from build123d import *

# Parameters (mm, degrees)
SCHIZZO1_R                           = 4
ESTRUSIONE_ESTRUSIONE1_DEPTH         = 8
SVUOTA1_T                            = -2
ESTRUSIONE_ESTRUSIONE3_DEPTH         = 2
TAGLIO_ESTRUSIONE2_REACH             = 21.653
SCHIZZO4_R                           = 1
TAGLIO_ESTRUSIONE1_REACH             = 21.653
SCHIZZO2_R                           = 1.5
TAGLIO_ESTRUSIONE1_DIRECTION_2_DEPTH = 10


with BuildPart() as part:
    # Schizzo1 → Estrusione-Estrusione1 (new body)
    with BuildSketch(Plane.XY):
        Circle(SCHIZZO1_R)
    extrude(amount=ESTRUSIONE_ESTRUSIONE1_DEPTH)

    # Svuota1
    svuota1_openings = [part.faces().sort_by_distance(p)[0] for p in [
        (0, 0, 8),
    ]]
    offset(amount=SVUOTA1_T, openings=svuota1_openings, kind=Kind.INTERSECTION)

    # Schizzo5 → Estrusione-Estrusione3 (add)
    with BuildSketch(Plane(origin=(0, 0, 0), x_dir=(-1, 0, 0), z_dir=(0, 0, -1))):
        with BuildLine():
            ThreePointArc((-3.920792079, 0.792079208), (0, 4), (3.920792079, 0.792079208))
            Line((3.920792079, 0.792079208), (2.5, 15))
            ThreePointArc((2.5, 15), (0, 17.5), (-2.5, 15))
            Line((-2.5, 15), (-3.920792079, 0.792079208))
        make_face()
    extrude(amount=-ESTRUSIONE_ESTRUSIONE3_DEPTH)

    # Schizzo4 → Taglio-Estrusione2 (cut, up to next)
    with BuildSketch(Plane(origin=(0, 0, 0), x_dir=(-1, 0, 0), z_dir=(0, 0, -1)), mode=Mode.PRIVATE) as taglio_estrusione2_sk1:
        with Locations((0, 6)):
            Circle(SCHIZZO4_R)
    taglio_estrusione2_tool1 = extrude(taglio_estrusione2_sk1.sketch, amount=-TAGLIO_ESTRUSIONE2_REACH, mode=Mode.PRIVATE) & part.part
    # Schizzo4 → Taglio-Estrusione2 (cut, up to next)
    with BuildSketch(Plane(origin=(0, 0, 0), x_dir=(-1, 0, 0), z_dir=(0, 0, -1)), mode=Mode.PRIVATE) as taglio_estrusione2_sk2:
        with Locations((0, 9)):
            Circle(SCHIZZO4_R)
    taglio_estrusione2_tool2 = extrude(taglio_estrusione2_sk2.sketch, amount=-TAGLIO_ESTRUSIONE2_REACH, mode=Mode.PRIVATE) & part.part
    # Schizzo4 → Taglio-Estrusione2 (cut, up to next)
    with BuildSketch(Plane(origin=(0, 0, 0), x_dir=(-1, 0, 0), z_dir=(0, 0, -1)), mode=Mode.PRIVATE) as taglio_estrusione2_sk3:
        with Locations((0, 12)):
            Circle(SCHIZZO4_R)
    taglio_estrusione2_tool3 = extrude(taglio_estrusione2_sk3.sketch, amount=-TAGLIO_ESTRUSIONE2_REACH, mode=Mode.PRIVATE) & part.part
    # Schizzo4 → Taglio-Estrusione2 (cut, up to next)
    with BuildSketch(Plane(origin=(0, 0, 0), x_dir=(-1, 0, 0), z_dir=(0, 0, -1)), mode=Mode.PRIVATE) as taglio_estrusione2_sk4:
        with Locations((0, 15)):
            Circle(SCHIZZO4_R)
    taglio_estrusione2_tool4 = extrude(taglio_estrusione2_sk4.sketch, amount=-TAGLIO_ESTRUSIONE2_REACH, mode=Mode.PRIVATE) & part.part
    add(taglio_estrusione2_tool1.solids().sort_by_distance((0, 6, 0))[0], mode=Mode.SUBTRACT)
    add(taglio_estrusione2_tool2.solids().sort_by_distance((0, 9, 0))[0], mode=Mode.SUBTRACT)
    add(taglio_estrusione2_tool3.solids().sort_by_distance((0, 12, 0))[0], mode=Mode.SUBTRACT)
    add(taglio_estrusione2_tool4.solids().sort_by_distance((0, 15, 0))[0], mode=Mode.SUBTRACT)

    # Schizzo2 → Taglio-Estrusione1 (cut, up to next)
    with BuildSketch(Plane(origin=(0, 0, 0), x_dir=(-1, 0, 0), z_dir=(0, 0, -1)), mode=Mode.PRIVATE) as taglio_estrusione1_sk1:
        with Locations(Location((0, 0, 0), (0, 0, 180))):
            Circle(SCHIZZO2_R)
    taglio_estrusione1_tool1 = extrude(taglio_estrusione1_sk1.sketch, amount=-TAGLIO_ESTRUSIONE1_REACH, mode=Mode.PRIVATE) & part.part
    add(taglio_estrusione1_tool1.solids().sort_by_distance((0, 0, 0))[0], mode=Mode.SUBTRACT)

    # Schizzo2 → Taglio-Estrusione1 direction 2 (cut)
    with BuildSketch(Plane(origin=(0, 0, 0), x_dir=(-1, 0, 0), z_dir=(0, 0, -1))):
        with Locations(Location((0, 0, 0), (0, 0, 180))):
            Circle(SCHIZZO2_R)
    extrude(amount=TAGLIO_ESTRUSIONE1_DIRECTION_2_DEPTH, mode=Mode.SUBTRACT)


solid = part.part
The model under review builds one solid part; all positions refer to its coordinate system, in mm. A direction names the side the tool comes from. Give positions to 0.01 mm unless a question says otherwise; leave off trailing zeros. Write each loop counter-clockwise with the first axis right and the second up, starting at its lowest first coordinate (ties: lowest second). Pieces come first, ordered by that corner, then holes.
1. Wall thickness on L1, parallel to Y at x = 0, z = 1.45; L2, parallel to Y at x = 0, z = 6.8; L3, parallel to Z at x = -1.25, y = 6: over which ranges is each line inside the solid? List them lowest first.
2. Add section C-C, the plane z = 6.75. Write out the cut boundary in (x, y), plus the area to 3 significant figures.
3. Add section D-D, the plane y = 0. Write out the cut boundary in (x, z), plus the area to 3 significant figures.
4. Add section A-A, the plane y = 6. Write out the cut boundary in (x, z).
5. For P1, Ø1.5, axis at x = 1, z = 4.5, coming from the -Y side; P2, Ø1.8, axis at x = 0, y = 0, coming from the -Z side; P3, Ø4, axis at x = 1.5, y = 11, coming from the +Z side; P4, Ø4, axis at x = 2.5, z = 2.5, coming from the +Y side, all flat-tipped, find the tip position at first contact; note any pin that passes through.
6. Add section B-B, the plane z = 1. Write out the cut boundary in (x, y).
7. Tool access review of faces 1 (the cylindrical face through (0, -2, 5)), 2 (the cylindrical face through (1.43, -0.45, 0.99)): name each direction out of +Z, -Z, +X, -X, +Y, -Y from which nothing blocks a thin tool from reaching the whole face with its end or side.
8. Draft analysis for pull direction Y (two halves, no side actions). For faces 3 (the cylindrical face through (0, 14, 1)), 4 (the cylindrical face through (-0.1, 17.5, 1)), 5 (the cylindrical face through (-0.867, -3.905, 3.944)), 6 (the flat face through (-2, 9, 2)), state which applies: +Y half, -Y half, draft (parallel to the pull), parting line (faces both ways), or undercut.
Worked answers:
1. L1: y = -4 to -1.5, 1.5 to 5, 7 to 8, 10 to 11, 13 to 14, 16 to 17.5
1. L2: y = -4 to -2, 2 to 4
1. L3: z = 0 to 2
2. outline: circle Ø8 at (0, 0); hole circle Ø4 at (0, 0)
2. area: 37.7 mm2
3. outline: (-4, 0) - (-1.5, 0) - (-1.5, 2) - (-2, 2) - (-2, 8) - (-4, 8) - close; (1.5, 0) - (4, 0) - (4, 8) - (2, 8) - (2, 2) - (1.5, 2) - close
3. area: 34.0 mm2
4. outline: (-3.4, 0) - (-1, 0) - (-1, 2) - (-3.4, 2) - close; (1, 0) - (3.4, 0) - (3.4, 2) - (1, 2) - close
5. P1: stops at y = -3.99
5. P2: passes through
5. P3: stops at z = 2
5. P4: stops at y = 17.44
6. outline: (-3.92, 0.79) arc R4 ccw (long way) to (3.92, 0.79) - (2.5, 15) arc R2.5 ccw to (-2.5, 15) - close; hole circle Ø3 at (0, 0); hole circle Ø2 at (0, 6); hole circle Ø2 at (0, 9); hole circle Ø2 at (0, 12); hole circle Ø2 at (0, 15)
7. face 1: +Z
7. face 2: +Z, -Z
8. face 3: undercut
8. face 4: +Y half
8. face 5: parting line
8. face 6: draft
